Autodesk Inventor part; units mm, degrees
ref_plane "YZ Plane" through (0, 0, 0) normal (1, 0, 0) x (0, 1, 0)
ref_plane "XZ Plane" through (0, 0, 0) normal (0, 1, 0) x (-1, 0, 0)
ref_plane "XY Plane" through (0, 0, 0) normal (0, 0, 1) x (1, 0, 0)
sketch "Sketch1" plane through (0, 0, 0) normal (0, 1, 0) x (-1, 0, 0)
  line L0 (7.5, 80) -> (-7.5, 80)
  line L1 (-7.5, -80) -> (7.5, -80)
  line L2 (7.5, 75.75) -> (9, 75.75)
  line L3 (7.5, 80) -> (9, 80)
  line L4 (7.5, 71.5) -> (9, 71.5)
  arc A0 (9, 71.5) -> (9, 80) centre (9, 75.75) ccw
  line L5 (7.5, 74.6) -> (9, 74.6)
  line L6 (7.5, 76.9) -> (9, 76.9)
  arc A1 (9, 74.6) -> (9, 76.9) centre (9, 75.75) ccw
  line L7 (-7.5, 80) -> (-9, 80)
  line L8 (-7.5, 71.5) -> (-9, 71.5)
  arc A2 (-9, 80) -> (-9, 71.5) centre (-9, 75.75) ccw
  line L9 (-7.5, 74.6) -> (-9, 74.6)
  line L10 (-7.5, 76.9) -> (-9, 76.9)
  arc A3 (-9, 76.9) -> (-9, 74.6) centre (-9, 75.75) ccw
  line L11 (7.5, -80) -> (9, -80)
  line L12 (7.5, -71.5) -> (9, -71.5)
  arc A4 (9, -80) -> (9, -71.5) centre (9, -75.75) ccw
  line L13 (7.5, -74.6) -> (9, -74.6)
  line L14 (7.5, -76.9) -> (9, -76.9)
  arc A5 (9, -76.9) -> (9, -74.6) centre (9, -75.75) ccw
  arc A6 (-9, -71.5) -> (-9, -80) centre (-9, -75.75) ccw
  line L15 (-7.5, -71.5) -> (-9, -71.5)
  line L16 (-7.5, -74.6) -> (-9, -74.6)
  arc A7 (-9, -74.6) -> (-9, -76.9) centre (-9, -75.75) ccw
  line L17 (-7.5, -76.9) -> (-9, -76.9)
  line L18 (-7.5, -80) -> (-9, -80)
  line L19 (7.5, 55) -> (27.5, 55)
  line L20 (32.5, 50) -> (32.5, 30)
  line L21 (32.5, 30) -> (42.5, 30)
  line L22 (47.5, 25) -> (47.5, 0)
  line L23 (7.5, -55) -> (27.5, -55)
  line L24 (32.5, -50) -> (32.5, -30)
  line L25 (32.5, -30) -> (42.5, -30)
  line L26 (47.5, -25) -> (47.5, 0)
  line L27 (27.5, 55) -> (32.5, 50)
  line L28 (42.5, 30) -> (47.5, 25)
  line L29 (47.5, -25) -> (42.5, -30)
  line L30 (32.5, -50) -> (27.5, -55)
  circle A8 centre (40.5, 0) radius 1.025
  circle A9 centre (-11.5, 0) radius 1.025
  line L31 (-7.5, 2.5) -> (-13.5, 2.5)
  line L32 (-13.5, 2.5) -> (-13.5, -2.5)
  line L33 (-13.5, -2.5) -> (-7.5, -2.5)
  line L34 (-12.525, 0) -> (-13.5, 0) construction
  line L35 (7.5, 55) -> (7.5, 71.5)
  line L36 (7.5, 74.6) -> (7.5, 76.9)
  line L37 (-7.5, 76.9) -> (-7.5, 74.6)
  line L38 (-7.5, 71.5) -> (-7.5, 2.5)
  line L39 (7.5, -76.9) -> (7.5, -74.6)
  line L40 (7.5, -71.5) -> (7.5, -55)
  line L41 (-7.5, -2.5) -> (-7.5, -71.5)
  line L42 (-7.5, -74.6) -> (-7.5, -76.9)
  point P0 (8.25, 71.5)
  point P1 (32.5, 55)
  point P2 (47.5, 30)
  point P3 (32.5, -55)
  point P4 (47.5, -30)
  dimension "d26" = 2.05
  dimension "d0" = 160
  dimension "d2" = 1.5
  dimension "d3" = 4.25
  dimension "d5" = 4.25
  dimension "d6" = 4.25
  dimension "d7" = 1.15
  dimension "d8" = 1.15
  dimension "d9" = 1.15
  dimension "d10" = 25
  dimension "d11" = 25
  dimension "d12" = 15
  dimension "d13" = 25
  dimension "d14" = 25
  dimension "d15" = 5
  dimension "d16" = 5
  dimension "d17" = 5
  dimension "d18" = 5
  dimension "d19" = 5
  dimension "d20" = 5
  dimension "d21" = 5
  dimension "d22" = 5
  dimension "d24" = 2.05
  dimension "d25" = 7
extrude "Extrusion1" add sketch "Sketch1" along normal blind 1.5 contours L3 A0 L4 L35 L19 L27 L20 L21 L28 L22 L26 L29 L25 L24 L30 L23 L40 L12 A4 L11 L1 L18 A6 L15 L41 L33 L32 L31 L38 L8 A2 L7 L0 | L36 L6 A1 L5 | L42 L17 A7 L16 | A9
properties part number "linefollower_chassy_model_3"
Geometry check sheet. Reference: the model listing, model coordinates, mm. Coordinates: 2 decimals unless noted, no trailing zeros. Order: outer loops, then holes, each group sorted by start corner. A loop starts at its lowest first (then second) coordinate and runs counter-clockwise, first axis right, second up.
Q1. Depth check by flat-ended pin: pin 1 Ø3.5 at (x, z) = (-40.5, 0) entering from +Y; pin 2 Ø0.8 at (y, z) = (1, -76) entering from -X. Enter the tip coordinate at first touch or a pass-through.
Reply:
pin 1: stops at y = 1.5
pin 2: stops at x = -13.25
Q2. Draft check along Z on faces 1 (the face through (-17, 1.5, 1)), 2 (the face through (-30, 0.7, -52.5)), 3 (the face through (13.25, 0.74, -75.84)). Enter one of: released by +Z, released by -Z, zero draft, split by the parting line, or undercut.
Reply:
face 1: zero draft
face 2: released by -Z
face 3: undercut
Q3. Thickness scan on probe 1 along Z at (x, y) = (8, 0.2); probe 2 along Z at (x, y) = (-40.5, 0.9) (3 decimals); probe 3 along Z at (x, y) = (10, 0.65). Record the ranges inside material, lowest first.
Reply:
probe 1: z = -80 to -71.5, -2.5 to 2.5, 71.5 to 74.6, 76.9 to 80
probe 2: z = -30 to -1.025, 1.025 to 30
probe 3: z = -79.88 to -71.62, -2.5 to 2.5, 71.62 to 75.18, 76.32 to 79.88
Q4. Sectioned sample at C-C on z = -27.5. Record the cut outline in (x, y).
Reply:
outline: (-45, 0) - (7.5, 0) - (7.5, 1.5) - (-45, 1.5) - close
Q5. Sectioned sample at A-A on y = 0.25. Give the number of separate pieces and of enclosed holes in the cut face, and give its area (3 significant figures).
Reply:
separate pieces: 1
enclosed holes: 3
area: 6,180 mm2
Q6. Sectioned sample at B-B on x = -20. Record the cut outline in (y, z).
Reply:
outline: (0, -55) - (1.5, -55) - (1.5, 55) - (0, 55) - close
